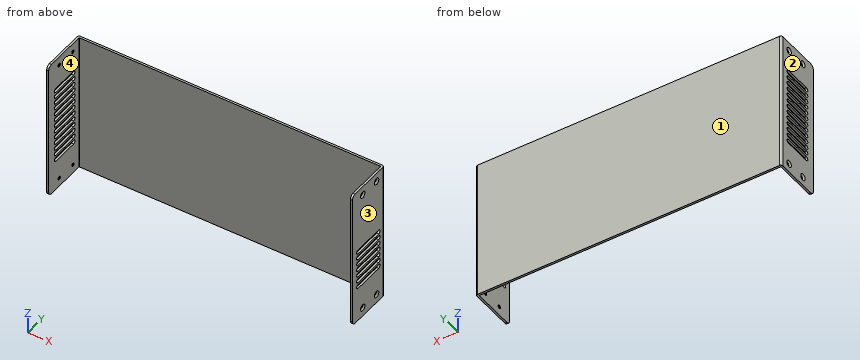
from build123d import *

# Parameters (mm, degrees)
BOSS_EXTRUDE1_DEPTH                             = 135
CSK_FOR_M3_FLAT_HEAD_MACHINE_SCREW1_D           = 3.4
CSK_FOR_M3_FLAT_HEAD_MACHINE_SCREW1_DEPTH       = 5
CSK_FOR_M3_FLAT_HEAD_MACHINE_SCREW1_CSINK_D     = 6.3
CSK_FOR_M3_FLAT_HEAD_MACHINE_SCREW1_CSINK_ANGLE = 90
CSK_FOR_M3_FLAT_HEAD_MACHINE_SCREW1_TIP         = 1.021463052
CSK_FOR_M3_FLAT_HEAD_MACHINE_SCREW2_D           = 3.4
CSK_FOR_M3_FLAT_HEAD_MACHINE_SCREW2_DEPTH       = 5
CSK_FOR_M3_FLAT_HEAD_MACHINE_SCREW2_CSINK_D     = 6.3
CSK_FOR_M3_FLAT_HEAD_MACHINE_SCREW2_CSINK_ANGLE = 90
CSK_FOR_M3_FLAT_HEAD_MACHINE_SCREW2_TIP         = 1.021463052
FILLET1_R                                       = 4
CUT_EXTRUDE1_DEPTH                              = 10
LPATTERN1_COUNT                                 = 13
LPATTERN1_PITCH                                 = 6
CUT_EXTRUDE2_DEPTH                              = 10
LPATTERN2_COUNT                                 = 7
LPATTERN2_PITCH                                 = 6


with BuildPart() as part:
    # Sketch1 → Boss-Extrude1 (new body)
    with BuildSketch(Plane.XY):
        with BuildLine():
            Line((0, 0), (-2, 0))
            Line((-2, 0), (-2, 44.2))
            ThreePointArc((-2, 44.2), (-1.472792206, 45.472792206), (-0.2, 46))
            Line((-0.2, 46), (290.2, 46))
            ThreePointArc((290.2, 46), (291.472792206, 45.472792206), (292, 44.2))
            Line((292, 44.2), (292, 0))
            Line((292, 0), (290, 0))
            Line((290, 0), (290, 43.5))
            ThreePointArc((290, 43.5), (289.853553391, 43.853553391), (289.5, 44))
            Line((289.5, 44), (0.5, 44))
            ThreePointArc((0.5, 44), (0.146446609, 43.853553391), (0, 43.5))
            Line((0, 43.5), (0, 0))
        make_face()
    extrude(amount=BOSS_EXTRUDE1_DEPTH)

    # CSK for M3 Flat Head Machine Screw1
    with Locations(Plane.ZY.offset(2)):
        with Locations((8.5, 35), (8.5, 15), (126.5, 35), (126.5, 15)):
            CounterSinkHole(CSK_FOR_M3_FLAT_HEAD_MACHINE_SCREW1_D / 2, CSK_FOR_M3_FLAT_HEAD_MACHINE_SCREW1_CSINK_D / 2, depth=CSK_FOR_M3_FLAT_HEAD_MACHINE_SCREW1_DEPTH, counter_sink_angle=CSK_FOR_M3_FLAT_HEAD_MACHINE_SCREW1_CSINK_ANGLE)
            with Locations((0, 0, -(CSK_FOR_M3_FLAT_HEAD_MACHINE_SCREW1_DEPTH + CSK_FOR_M3_FLAT_HEAD_MACHINE_SCREW1_TIP / 2))):  # 118° drill point
                Cone(0, CSK_FOR_M3_FLAT_HEAD_MACHINE_SCREW1_D / 2, CSK_FOR_M3_FLAT_HEAD_MACHINE_SCREW1_TIP, mode=Mode.SUBTRACT)

    # CSK for M3 Flat Head Machine Screw2
    with Locations(Plane(origin=(292, 0, 0), x_dir=(0, 0, -1), z_dir=(1, 0, 0))):
        with Locations((-126.5, 35), (-126.5, 15), (-8.5, 35), (-8.5, 15)):
            CounterSinkHole(CSK_FOR_M3_FLAT_HEAD_MACHINE_SCREW2_D / 2, CSK_FOR_M3_FLAT_HEAD_MACHINE_SCREW2_CSINK_D / 2, depth=CSK_FOR_M3_FLAT_HEAD_MACHINE_SCREW2_DEPTH, counter_sink_angle=CSK_FOR_M3_FLAT_HEAD_MACHINE_SCREW2_CSINK_ANGLE)
            with Locations((0, 0, -(CSK_FOR_M3_FLAT_HEAD_MACHINE_SCREW2_DEPTH + CSK_FOR_M3_FLAT_HEAD_MACHINE_SCREW2_TIP / 2))):  # 118° drill point
                Cone(0, CSK_FOR_M3_FLAT_HEAD_MACHINE_SCREW2_D / 2, CSK_FOR_M3_FLAT_HEAD_MACHINE_SCREW2_TIP, mode=Mode.SUBTRACT)

    # Fillet1
    fillet1_edges = [part.edges().sort_by_distance(p)[0] for p in [
        (-1, 0, 0),
        (291, 0, 0),
        (291, 0, 135),
        (-1, 0, 135),
    ]]
    fillet(fillet1_edges, radius=FILLET1_R)

    # Sketch6 → Cut-Extrude1 (cut)
    with BuildSketch(Plane(origin=(-2, 0, 0), x_dir=(0, 0, -1), z_dir=(1, 0, 0))):
        with BuildLine():
            Line((-101.5, 36), (-101.5, 10))
            ThreePointArc((-101.5, 10), (-103.5, 8), (-105.5, 10))
            Line((-105.5, 10), (-105.5, 36))
            ThreePointArc((-105.5, 36), (-103.5, 38), (-101.5, 36))
        make_face()
    cut_extrude1 = extrude(amount=CUT_EXTRUDE1_DEPTH, mode=Mode.SUBTRACT)

    # LPattern1: Cut-Extrude1 ×13
    with Locations(*[(0, 0, -i * LPATTERN1_PITCH) for i in range(1, LPATTERN1_COUNT)]):
        add(cut_extrude1, mode=Mode.SUBTRACT)

    # Sketch7 → Cut-Extrude2 (cut)
    with BuildSketch(Plane(origin=(292, 0, 0), x_dir=(0, 0, -1), z_dir=(1, 0, 0))):
        with BuildLine():
            Line((-33.5, 38), (-33.5, 8))
            ThreePointArc((-33.5, 8), (-35.5, 6), (-37.5, 8))
            Line((-37.5, 8), (-37.5, 38))
            ThreePointArc((-37.5, 38), (-35.5, 40), (-33.5, 38))
        make_face()
    cut_extrude2 = extrude(amount=-CUT_EXTRUDE2_DEPTH, mode=Mode.SUBTRACT)

    # LPattern2: Cut-Extrude2 ×7
    with Locations(*[(0, 0, i * LPATTERN2_PITCH) for i in range(1, LPATTERN2_COUNT)]):
        add(cut_extrude2, mode=Mode.SUBTRACT)


solid = part.part
Could you check a few things on this model? Use its own coordinates, in mm. Face numbers are marked on the shaded views. Give positions to 0.01 mm unless a question says otherwise; leave off trailing zeros. Order: outer loops, then holes, each group sorted by start corner. A loop starts at its lowest first (then second) coordinate and runs counter-clockwise, first axis right, second up. Notation, with made-up numbers: (47.5, -36) -> (57.5, -36) arc R24 ccw to (57.5, -7) -> close; hole circle Ø2 at (-9.5, 15.5). An arc over 180 degrees is marked (long way). Answer in a Markdown table with one row per item. Add a question column.
Item 1: We'd pull the mould along X, two halves only. Please class the marked faces 1, 2, 3 and 4: pulls with the +X half, pulls with the -X half, needs draft (parallel to the pull), parting line crosses it, or undercut.
Item 2: Imagine slicing it at B-B (x = 100.5). List the corners of the cut face in (y, z) for me.
Item 3: I'm going to push flat-ended pins straight in: P1, Ø4, axis at y = 35, z = 8.5, coming from the -X side; P2, Ø10, axis at x = 131.5, z = 77.5, coming from the -Y side; P3, Ø4.5, axis at y = 15, z = 126.5, coming from the -X side. Where does each tip first touch, or does it pass through?
Item 4: Please list where these lines run through material, in increasing order: probe 1 along Y at (x, z) = (290.15, 8.5); probe 2 along X at (y, z) = (2, 65); probe 3 along X at (y, z) = (17, 59).
Item 5: Imagine slicing it at A-A (y = 25). Count the separate pieces of the cut face and the enclosed holes in it, and give its area (3 significant figures).
Result:
| question | item | result |
|---|---|---|
| 1 | face 1 | needs draft |
| 1 | face 2 | pulls with the -X half |
| 1 | face 3 | pulls with the +X half |
| 1 | face 4 | undercut |
| 2 | outline | (44, 0) -> (46, 0) -> (46, 135) -> (44, 135) -> close |
| 3 | P1 | x = -0.85 |
| 3 | P2 | y = 44 |
| 3 | P3 | x = -1.1 |
| 4 | probe 1 | 0 to 13.3, 16.7 to 33.3, 36.7 to 46 |
| 4 | probe 2 | -2 to 0, 290 to 292 |
| 4 | probe 3 | -2 to 0 |
| 5 | separate pieces | 22 |
| 5 | enclosed holes | 0 |
| 5 | area | 380 mm2 |
